Geometry: final body of the model. Coordinates: model frame, mm. Coordinates: 2 decimals unless noted, no trailing zeros. Write each loop counter-clockwise with the first axis right and the second up, starting at its lowest first coordinate (ties: lowest second). Pieces come first, ordered by that corner, then holes. Notation, with made-up numbers: (20, -22.5) - (59, -22.5) arc R20 ccw to (59, 12.5) - close; hole circle Ø1 at (73.5, 87.25). An arc over 180 degrees is marked (long way). Put each result on its own line as item: value.
```python
from build123d import *

# Parameters (mm, degrees)
ESTRUSIONE_ESTRUSIONE1_DEPTH = 18
TAGLIO_ESTRUSIONE1_DEPTH     = 47
TAGLIO_ESTRUSIONE2_DEPTH     = 32
TAGLIO_ESTRUSIONE3_DEPTH     = 50
TAGLIO_ESTRUSIONE4_DEPTH     = 44
TAGLIO_ESTRUSIONE5_DEPTH     = 38
TAGLIO_ESTRUSIONE6_DEPTH     = 44
MODEL_11_R                   = 186.766541562
TAGLIO_ESTRUSIONE7_DEPTH     = 91


with BuildPart() as part:
    # Model → Estrusione-Estrusione1 (new body)
    with BuildSketch(Plane.XY):
        with BuildLine():
            Line((-275, -232), (-275, 232))
            Line((-275, 232), (-231.35, 232))
            ThreePointArc((-231.35, 232), (-228.175, 228.825), (-225, 232))
            Line((-225, 232), (-225, 250))
            Line((-225, 250), (-175, 250))
            Line((-175, 250), (-175, 232))
            ThreePointArc((-175, 232), (-171.825, 228.825), (-168.65, 232))
            Line((-168.65, 232), (-131.35, 232))
            ThreePointArc((-131.35, 232), (-128.175, 228.825), (-125, 232))
            Line((-125, 232), (-125, 250))
            Line((-125, 250), (-75, 250))
            Line((-75, 250), (-75, 232))
            ThreePointArc((-75, 232), (-71.825, 228.825), (-68.65, 232))
            Line((-68.65, 232), (-31.35, 232))
            ThreePointArc((-31.35, 232), (-28.175, 228.825), (-25, 232))
            Line((-25, 232), (-25, 250))
            Line((-25, 250), (25, 250))
            Line((25, 250), (25, 232))
            ThreePointArc((25, 232), (28.175, 228.825), (31.35, 232))
            Line((31.35, 232), (68.65, 232))
            ThreePointArc((68.65, 232), (71.825, 228.825), (75, 232))
            Line((75, 232), (75, 250))
            Line((75, 250), (125, 250))
            Line((125, 250), (125, 232))
            ThreePointArc((125, 232), (128.175, 228.825), (131.35, 232))
            Line((131.35, 232), (168.65, 232))
            ThreePointArc((168.65, 232), (171.825, 228.825), (175, 232))
            Line((175, 232), (175, 250))
            Line((175, 250), (225, 250))
            Line((225, 250), (225, 232))
            ThreePointArc((225, 232), (228.175, 228.825), (231.35, 232))
            Line((231.35, 232), (275, 232))
            Line((275, 232), (275, -232))
            Line((275, -232), (231.35, -232))
            ThreePointArc((231.35, -232), (228.175, -228.825), (225, -232))
            Line((225, -232), (225, -250))
            Line((225, -250), (175, -250))
            Line((175, -250), (175, -232))
            ThreePointArc((175, -232), (171.825, -228.825), (168.65, -232))
            Line((168.65, -232), (131.35, -232))
            ThreePointArc((131.35, -232), (128.175, -228.825), (125, -232))
            Line((125, -232), (125, -250))
            Line((125, -250), (75, -250))
            Line((75, -250), (75, -232))
            ThreePointArc((75, -232), (71.825, -228.825), (68.65, -232))
            Line((68.65, -232), (31.35, -232))
            ThreePointArc((31.35, -232), (28.175, -228.825), (25, -232))
            Line((25, -232), (25, -250))
            Line((25, -250), (-25, -250))
            Line((-25, -250), (-25, -232))
            ThreePointArc((-25, -232), (-28.175, -228.825), (-31.35, -232))
            Line((-31.35, -232), (-68.65, -232))
            ThreePointArc((-68.65, -232), (-71.825, -228.825), (-75, -232))
            Line((-75, -232), (-75, -250))
            Line((-75, -250), (-125, -250))
            Line((-125, -250), (-125, -232))
            ThreePointArc((-125, -232), (-128.175, -228.825), (-131.35, -232))
            Line((-131.35, -232), (-168.65, -232))
            ThreePointArc((-168.65, -232), (-171.825, -228.825), (-175, -232))
            Line((-175, -232), (-175, -250))
            Line((-175, -250), (-225, -250))
            Line((-225, -250), (-225, -232))
            ThreePointArc((-225, -232), (-228.175, -228.825), (-231.35, -232))
            Line((-231.35, -232), (-275, -232))
        make_face()
    extrude(amount=ESTRUSIONE_ESTRUSIONE1_DEPTH)

    # Model_3 → Taglio-Estrusione1 (cut)
    with BuildSketch(Plane.XY):
        with BuildLine():
            Line((-255, 145.65), (-255, 108.35))
            ThreePointArc((-255, 108.35), (-258.175, 105.175), (-255, 102))
            Line((-255, 102), (-237, 102))
            ThreePointArc((-237, 102), (-233.825, 105.175), (-237, 108.35))
            Line((-237, 108.35), (-237, 145.65))
            ThreePointArc((-237, 145.65), (-233.825, 148.825), (-237, 152))
            Line((-237, 152), (-255, 152))
            ThreePointArc((-255, 152), (-258.175, 148.825), (-255, 145.65))
        make_face()
    extrude(amount=TAGLIO_ESTRUSIONE1_DEPTH, mode=Mode.SUBTRACT)

    # Model_4 → Taglio-Estrusione2 (cut)
    with BuildSketch(Plane.XY):
        with BuildLine():
            Line((-255, -18.65), (-255, 18.65))
            ThreePointArc((-255, 18.65), (-258.175, 21.825), (-255, 25))
            Line((-255, 25), (-237, 25))
            ThreePointArc((-237, 25), (-233.825, 21.825), (-237, 18.65))
            Line((-237, 18.65), (-237, -18.65))
            ThreePointArc((-237, -18.65), (-233.825, -21.825), (-237, -25))
            Line((-237, -25), (-255, -25))
            ThreePointArc((-255, -25), (-258.175, -21.825), (-255, -18.65))
        make_face()
    extrude(amount=TAGLIO_ESTRUSIONE2_DEPTH, mode=Mode.SUBTRACT)

    # Model_5 → Taglio-Estrusione3 (cut)
    with BuildSketch(Plane.XY):
        with BuildLine():
            Line((-255, -145.65), (-255, -108.35))
            ThreePointArc((-255, -108.35), (-258.175, -105.175), (-255, -102))
            Line((-255, -102), (-237, -102))
            ThreePointArc((-237, -102), (-233.825, -105.175), (-237, -108.35))
            Line((-237, -108.35), (-237, -145.65))
            ThreePointArc((-237, -145.65), (-233.825, -148.825), (-237, -152))
            Line((-237, -152), (-255, -152))
            ThreePointArc((-255, -152), (-258.175, -148.825), (-255, -145.65))
        make_face()
    extrude(amount=TAGLIO_ESTRUSIONE3_DEPTH, mode=Mode.SUBTRACT)

    # Model_6 → Taglio-Estrusione4 (cut)
    with BuildSketch(Plane.XY):
        with BuildLine():
            Line((237, 145.65), (237, 108.35))
            ThreePointArc((237, 108.35), (233.825, 105.175), (237, 102))
            Line((237, 102), (255, 102))
            ThreePointArc((255, 102), (258.175, 105.175), (255, 108.35))
            Line((255, 108.35), (255, 145.65))
            ThreePointArc((255, 145.65), (258.175, 148.825), (255, 152))
            Line((255, 152), (237, 152))
            ThreePointArc((237, 152), (233.825, 148.825), (237, 145.65))
        make_face()
    extrude(amount=TAGLIO_ESTRUSIONE4_DEPTH, mode=Mode.SUBTRACT)

    # Model_7 → Taglio-Estrusione5 (cut)
    with BuildSketch(Plane.XY):
        with BuildLine():
            Line((237, -18.65), (237, 18.65))
            ThreePointArc((237, 18.65), (233.825, 21.825), (237, 25))
            Line((237, 25), (255, 25))
            ThreePointArc((255, 25), (258.175, 21.825), (255, 18.65))
            Line((255, 18.65), (255, -18.65))
            ThreePointArc((255, -18.65), (258.175, -21.825), (255, -25))
            Line((255, -25), (237, -25))
            ThreePointArc((237, -25), (233.825, -21.825), (237, -18.65))
        make_face()
    extrude(amount=TAGLIO_ESTRUSIONE5_DEPTH, mode=Mode.SUBTRACT)

    # Model_10 → Taglio-Estrusione6 (cut)
    with BuildSketch(Plane.XY):
        with BuildLine():
            Line((237, -145.65), (237, -108.35))
            ThreePointArc((237, -108.35), (233.825, -105.175), (237, -102))
            Line((237, -102), (255, -102))
            ThreePointArc((255, -102), (258.175, -105.175), (255, -108.35))
            Line((255, -108.35), (255, -145.65))
            ThreePointArc((255, -145.65), (258.175, -148.825), (255, -152))
            Line((255, -152), (237, -152))
            ThreePointArc((237, -152), (233.825, -148.825), (237, -145.65))
        make_face()
    extrude(amount=TAGLIO_ESTRUSIONE6_DEPTH, mode=Mode.SUBTRACT)

    # Model_11 → Taglio-Estrusione7 (cut)
    with BuildSketch(Plane.XY):
        with Locations(Location((0, 0, 0), (0, 0, 180))):
            Circle(MODEL_11_R)
    extrude(amount=TAGLIO_ESTRUSIONE7_DEPTH, mode=Mode.SUBTRACT)


solid = part.part
```
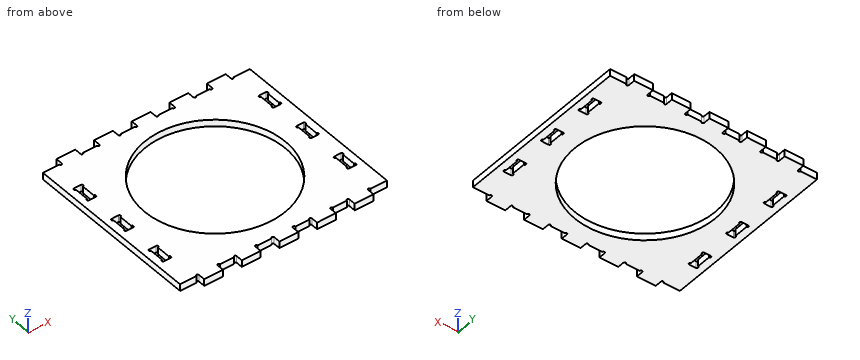
1. Section query D-D (z = 9). Count the separate pieces of the cut face and the enclosed holes in it, then the cut area to 3 significant figures.
Answer below:
separate pieces: 1
enclosed holes: 7
area: 149,000 mm²
2. Section query B-B (x = 0). Return loops of the section in (y, z), then the cut area to 3 significant figures.
Answer below:
outline: (-250, 0) - (-186.77, 0) - (-186.77, 18) - (-250, 18) - close; (186.77, 0) - (250, 0) - (250, 18) - (186.77, 18) - close
area: 2,280 mm²
3. Section query A-A (y = 0). Return loops of the section in (x, z), then the cut area to 3 significant figures.
Answer below:
outline: (-275, 0) - (-255, 0) - (-255, 18) - (-275, 18) - close; (-237, 0) - (-186.77, 0) - (-186.77, 18) - (-237, 18) - close; (186.77, 0) - (237, 0) - (237, 18) - (186.77, 18) - close; (255, 0) - (275, 0) - (275, 18) - (255, 18) - close
area: 2,530 mm²
4. Pin query (flat end, axial travel): pin 1 Ø9 at (x, z) = (242.5, 12.5) entering from +Y. Return the tip coordinate at first contact, or that it passes through.
Answer below:
pin 1: stops at y = 232
5. Ray query, probe 1 along X at (y, z) = (111.5, 6.75); probe 2 along X at (y, z) = (-143.5, 16.25); probe 3 along Y at (x, z) = (0, 8). Return the intervals inside material, ascending. Write a range as from..to.
Answer below:
probe 1: x = -275..-255, -237..-149.83, 149.83..237, 255..275
probe 2: x = -275..-255, -237..-119.54, 119.54..237, 255..275
probe 3: y = -250..-186.77, 186.77..250
6. Section query C-C (y = -55.5). Return loops of the section in (x, z).
Answer below:
outline: (-275, 0) - (-178.33, 0) - (-178.33, 18) - (-275, 18) - close; (178.33, 0) - (275, 0) - (275, 18) - (178.33, 18) - close
